```python
from build123d import *

# Parameters (mm, degrees)
F0_W     = 254
F0_H     = 152.4
F1_DEPTH = 63.5
F2_W     = 238.76
F2_H     = 111.76
F3_DEPTH = 114.3
F4_W     = 203.2
F4_H     = 101.6
F5_DEPTH = 25.4


with BuildPart() as f1:
    # F0 (on Front) → F1 (new body, symmetric)
    with BuildSketch(Plane.XZ):
        with Locations((9.614129, 15.851616)):
            Rectangle(F0_W, F0_H)
    extrude(amount=F1_DEPTH, both=True)

    # F2 (on face) → F3 (cut)
    with BuildSketch(Plane.XY.offset(92.051616)):
        with Locations((9.614129, 0)):
            Rectangle(F2_W, F2_H)
    extrude(amount=-F3_DEPTH, mode=Mode.SUBTRACT)

    # F4 (on face) → F5 (cut)
    with BuildSketch(Plane.XZ.offset(63.5)):
        with Locations((9.614129, 15.851616)):
            Rectangle(F4_W, F4_H)
    extrude(amount=-F5_DEPTH, mode=Mode.SUBTRACT)


solid = f1.part
```
Geometry: final body of the model. Coordinates: model frame, mm. A direction names the side the tool comes from. Round coordinates to 2 decimals unless told otherwise and drop trailing zeros. Order: outer loops, then holes, each group sorted by start corner. A loop starts at its lowest first (then second) coordinate and runs counter-clockwise, first axis right, second up. Notation, with made-up numbers: (-14.5, 62) - (42.5, 62) arc R25 cw to (42.5, 84) - close; hole circle Ø11 at (76, -22.5). An arc over 180 degrees is marked (long way). Write item = value, one per line. Start each with the question number.
Q1. Cut plane C-C on z = -29. Return the cut outline in (x, y).
Q2. Ray query, line 1 (Y direction, x = 66.5, z = 76); line 2 (X direction, y = 37.5, z = 48.5); line 3 (Z direction, x = -66.5, y = 22). Return the intervals inside material, ascending. Write a range as from..to.
Q3. Cut plane B-B on x = -1. Return the cut outline in (y, z), and give its area (3 significant figures).
Q4. Access query for faces 5 (the flat face through (8, -55.88, 74)), 6 (the flat face through (8, -63.5, 68)), 7 (the flat face through (8, -60, 66.652)). Directions: +Z, -Z, +X, -X, +Y, -Y. A direction counts if a zero-diameter tool reaches every point of the face in a straight line with its end or side. Return the directions, or none.
Q5. Pull-direction query (Y, two-part tool) for faces 1 (the flat face through (8, 55.88, 36)), 2 (the flat face through (-117.386, -1, 15)), 3 (the flat face through (8, -38.1, -29)), 4 (the flat face through (-109.766, -1, 36)); classes: +Y half, -Y half, draft (parallel to the pull), parting line (faces both ways), or undercut.
Q6. Cut plane D-D on x = 117. Return the cut outline in (y, z), and give its area (3 significant figures).
Q7. Cut plane A-A on z = 79. Return the cut outline in (x, y).
Q8. Pin query (flat end, axial travel): pin 1 (10 mm diameter, centred on x = 55, y = -47, fed in from +Z); pin 2 (1 mm diameter, centred on x = -87, z = 35.5, fed in from -Y); pin 3 (6.5 mm diameter, centred on x = -11, z = -26, fed in from -Y). Return the tip coordinate at first contact, or that it passes through.
Outcome:
q1.outline = (-117.39, -63.5) - (-91.99, -63.5) - (-91.99, -38.1) - (111.21, -38.1) - (111.21, -63.5) - (136.61, -63.5) - (136.61, 63.5) - (-117.39, 63.5) - close
q2.line_1 = -63.5..-55.88, 55.88..63.5
q2.line_2 = -117.39..-109.77, 128.99..136.61
q2.line_3 = -60.35..-22.25
q3.outline = (-63.5, -60.35) - (63.5, -60.35) - (63.5, 92.05) - (55.88, 92.05) - (55.88, -22.25) - (-38.1, -22.25) - (-38.1, -34.95) - (-63.5, -34.95) - close; (-63.5, 66.65) - (-55.88, 66.65) - (-55.88, 92.05) - (-63.5, 92.05) - close
q3.area = 5,580 mm^2
q4.face_5 = +Z
q4.face_6 = +Z, -Z, +X, -X, -Y
q4.face_7 = -Y
q5.face_1 = undercut
q5.face_2 = draft
q5.face_3 = -Y half
q5.face_4 = undercut
q6.outline = (-63.5, -60.35) - (63.5, -60.35) - (63.5, 92.05) - (55.88, 92.05) - (55.88, -22.25) - (-55.88, -22.25) - (-55.88, 92.05) - (-63.5, 92.05) - close
q6.area = 6,580 mm^2
q7.outline = (-117.39, -63.5) - (136.61, -63.5) - (136.61, 63.5) - (-117.39, 63.5) - close; hole (-109.77, -55.88) - (128.99, -55.88) - (128.99, 55.88) - (-109.77, 55.88) - close
q8.pin_1 = -34.95
q8.pin_2 = 55.88
q8.pin_3 = -38.1
